Can you work these out from the model? Positions are in its coordinate system, mm. Give positions to 0.01 mm unless a question says otherwise; leave off trailing zeros. Order: outer loops, then holes, each group sorted by start corner. A loop starts at its lowest first (then second) coordinate and runs counter-clockwise, first axis right, second up. Notation, with made-up numbers: (50.5, 27) - (85.5, 27) arc R11 ccw to (85.5, 36) - close; hole circle Ø9 at (4, 16.5). An arc over 180 degrees is marked (long way). Answer as CSV lines item,"result".
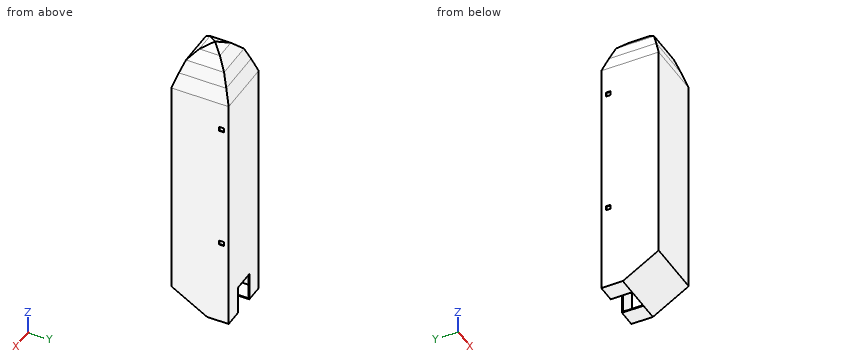
```python
from build123d import *

# Parameters (mm, degrees)
SKETCH1_W           = 101.6
SKETCH1_H           = 101.6
BOSS_EXTRUDE1_DEPTH = 436.88
SHELL1_T            = -1.5875
SKETCH9_W           = 8.001
SKETCH9_H           = 8.001
CUT_EXTRUDE1_DEPTH  = 526.503840631
CUT_EXTRUDE2_DEPTH  = 526.503840631
BOSS_EXTRUDE2_DEPTH = 101.6
SKETCH12_W          = 38.1
SKETCH12_H          = 38.1
CUT_EXTRUDE3_DEPTH  = 50.8


with BuildPart() as part:
    # Sketch1 → Boss-Extrude1 (new body)
    with BuildSketch(Plane.XY):
        Rectangle(SKETCH1_W, SKETCH1_H)
    extrude(amount=BOSS_EXTRUDE1_DEPTH)

    # Sketch5 → Loft2 section 0
    with BuildSketch(Plane.XY.offset(436.88)):
        with BuildLine():
            Line((50.8, -50.8), (50.8, 50.8))
            Line((50.8, 50.8), (-50.8, 50.8))
            Line((-50.8, 50.8), (-50.8, -50.8))
            Line((-50.8, -50.8), (50.8, -50.8))
        make_face()
    # Sketch3 → Loft2 section 1
    with BuildSketch(Plane.XY.offset(464.156588322)):
        with BuildLine():
            Line((-41.937305, -41.937305), (41.937305, -41.937305))
            Line((41.937305, -41.937305), (41.937305, 41.937305))
            Line((41.937305, 41.937305), (-41.937305, 41.937305))
            Line((-41.937305, 41.937305), (-41.937305, -41.937305))
        make_face()
    loft()

    # Sketch3_6 → Loft3 section 0
    with BuildSketch(Plane.XY.offset(464.156588322)):
        with BuildLine():
            Line((-41.937305, -41.937305), (41.937305, -41.937305))
            Line((41.937305, -41.937305), (41.937305, 41.937305))
            Line((41.937305, 41.937305), (-41.937305, 41.937305))
            Line((-41.937305, 41.937305), (-41.937305, -41.937305))
        make_face()
    # Sketch6 → Loft3 section 1
    with BuildSketch(Plane.XY.offset(487.359440316)):
        with BuildLine():
            Line((-33.71596, -33.71596), (33.71596, -33.71596))
            Line((33.71596, -33.71596), (33.71596, 33.71596))
            Line((33.71596, 33.71596), (-33.71596, 33.71596))
            Line((-33.71596, 33.71596), (-33.71596, -33.71596))
        make_face()
    loft()

    # Sketch6_4 → Loft4 section 0
    with BuildSketch(Plane.XY.offset(487.359440316)):
        with BuildLine():
            Line((-33.71596, -33.71596), (33.71596, -33.71596))
            Line((33.71596, -33.71596), (33.71596, 33.71596))
            Line((33.71596, 33.71596), (-33.71596, 33.71596))
            Line((-33.71596, 33.71596), (-33.71596, -33.71596))
        make_face()
    # Sketch7 → Loft4 section 1
    with BuildSketch(Plane.XY.offset(504.217299158)):
        with BuildLine():
            Line((-18.304143458, -18.304143458), (18.304143458, -18.304143458))
            Line((18.304143458, -18.304143458), (18.304143458, 18.304143458))
            Line((18.304143458, 18.304143458), (-18.304143458, 18.304143458))
            Line((-18.304143458, 18.304143458), (-18.304143458, -18.304143458))
        make_face()
    loft()

    # Sketch7_5 → Loft5 section 0
    with BuildSketch(Plane.XY.offset(504.217299158), mode=Mode.PRIVATE) as loft5_s0:
        with BuildLine():
            Line((-18.304143458, -18.304143458), (18.304143458, -18.304143458))
            Line((18.304143458, -18.304143458), (18.304143458, 18.304143458))
            Line((18.304143458, 18.304143458), (-18.304143458, 18.304143458))
            Line((-18.304143458, 18.304143458), (-18.304143458, -18.304143458))
        make_face()
    loft([Vertex(0, 0, 513.079999985), loft5_s0.sketch])

    # Shell1
    shell1_openings = [part.faces().sort_by_distance(p)[0] for p in [
        (0, 0, 0),
    ]]
    offset(amount=SHELL1_T, openings=shell1_openings, kind=Kind.INTERSECTION)

    # Sketch9 → Cut-Extrude1 (cut, through all)
    with BuildSketch(Plane(origin=(50.8, 0, 0), x_dir=(0, 0, -1), z_dir=(1, 0, 0))):
        with Locations((-386.08, 38.1)):
            Rectangle(SKETCH9_W, SKETCH9_H)
        with Locations((-157.48, 38.1)):
            Rectangle(SKETCH9_W, SKETCH9_H)
    extrude(amount=-CUT_EXTRUDE1_DEPTH, mode=Mode.SUBTRACT)

    # Sketch10 → Cut-Extrude2 (cut, through all)
    with BuildSketch(Plane(origin=(50.8, 0, 0), x_dir=(0, 0, -1), z_dir=(1, 0, 0))):
        Polygon((0, -50.8), (0, 12.7), (-38.1, -50.8), align=None)
    extrude(amount=-CUT_EXTRUDE2_DEPTH, mode=Mode.SUBTRACT)

    # Sketch11 → Boss-Extrude2 (add)
    with BuildSketch(Plane(origin=(50.8, 0, 0), x_dir=(0, 0, -1), z_dir=(1, 0, 0))):
        Polygon((-38.1, -50.8), (-39.6875, -50.8), (-1.5875, 12.7), (-1.5875, 50.8), (0, 50.8), (0, 12.7), align=None)
    extrude(amount=-BOSS_EXTRUDE2_DEPTH)

    # Sketch12 → Cut-Extrude3 (cut)
    with BuildSketch(Plane(origin=(0, 0, 0), x_dir=(-1, 0, 0), z_dir=(0, 0, -1))):
        with Locations((0, 31.75)):
            Rectangle(SKETCH12_W, SKETCH12_H)
    extrude(amount=-CUT_EXTRUDE3_DEPTH, mode=Mode.SUBTRACT)


solid = part.part
```
1) I'm going to push flat-ended pins straight in: P1, Ø24, axis at x = -39.5, y = 26, coming from the +Z side; P2, Ø5, axis at x = 33.5, y = 29.5, coming from the +Z side; P3, Ø0.5, axis at x = -50.5, y = 37, coming from the -Z side; P4, Ø15, axis at x = 40, y = 31.5, coming from the +Z side. Where does each tip first touch, or does it pass through?
Answer block:
P1,"z = 494.16"
P2,"z = 490.33"
P3,"z = 0"
P4,"z = 488.69"
2) I need wall thicknesses on line 1 along Y through (x, z) = (11.5, 364.5); line 2 along Y through (x, z) = (-18, 47). Which ranges of each line are inside material? Lowest first, please. Write a range as [from, to].
Answer block:
line 1,"[-50.8, -49.21], [49.21, 50.8]"
line 2,"[-50.8, -49.21]"
3) I want a section at A-A on z = 181. Write out the boundary of the cut face in (x, y).
Answer block:
outline,"(-50.8, -50.8) - (50.8, -50.8) - (50.8, 50.8) - (-50.8, 50.8) - close; hole (-49.21, -49.21) - (49.21, -49.21) - (49.21, 49.21) - (-49.21, 49.21) - close"
